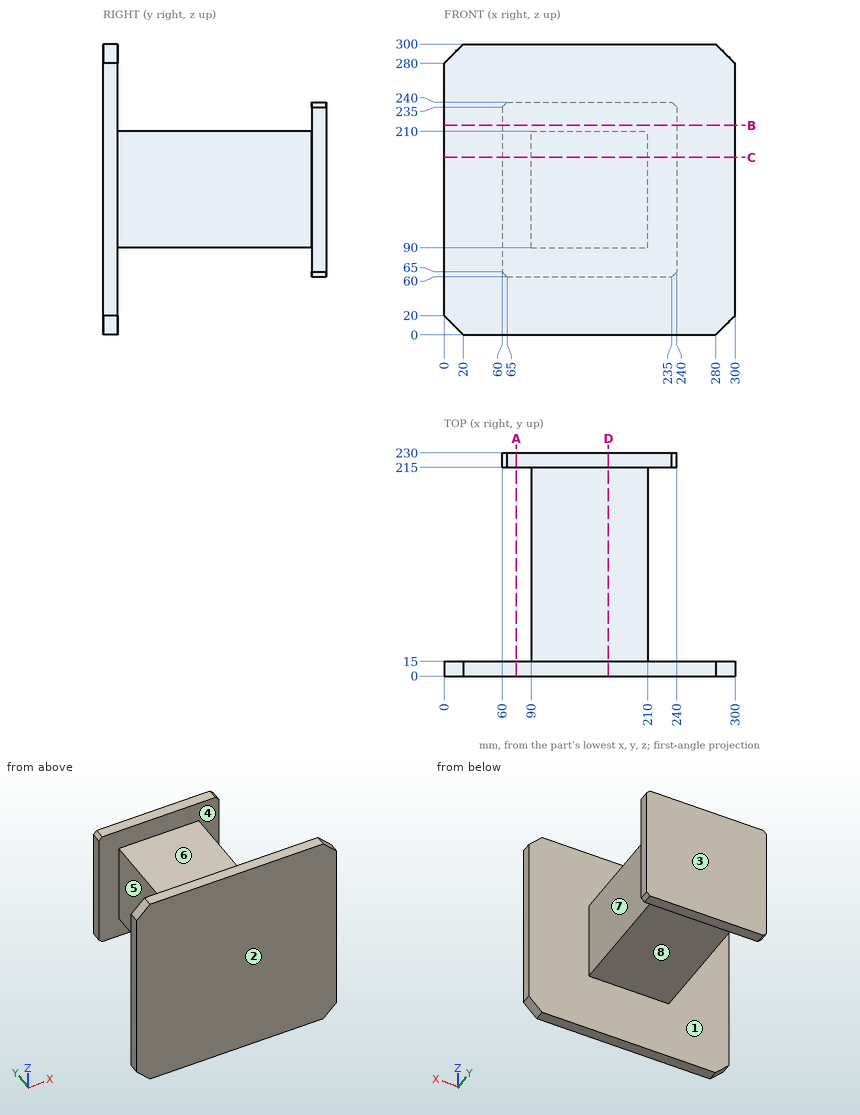
Print and shaded views of the part. All mm, measured from the part's lowest x, y and z. A direction names the side the tool comes from. Coordinates: 2 decimals unless noted, no trailing zeros. Order: outer loops, then holes, each group sorted by start corner. A loop starts at its lowest first (then second) coordinate and runs counter-clockwise, first axis right, second up. Notation, with made-up numbers: (42.25, 80.5) -> (60.25, 80.5) arc R25 ccw to (60.25, 102.5) -> close; hole circle Ø1 at (88.5, 73.5). An arc over 180 degrees is marked (long way). Answer as a JSON object with one key per item and string values. Group by question number.
1) Cut at B-B, the plane z = 216. Write the cut outline in (x, y).
2) Cut at C-C, the plane z = 183. Write the cut outline in (x, y).
3) Pull direction Y, two halves, no side cores. Call the marked faces 1, 2 and 3: +Y half, -Y half, draft (parallel to the pull), parting line (faces both ways), or undercut.
4) Flat gauge pins, fed straight in: pin 1 (3 mm diameter, centred on x = 190, y = 83.5, fed in from -Z); pin 2 (4.5 mm diameter, centred on y = 224.5, z = 182, fed in from +X); pin 3 (3 mm diameter, centred on y = 159, z = 203.5, fed in from +X); pin 4 (5 mm diameter, centred on x = 99.5, z = 88, fed in from -Y). Where does each tip first touch, or does it go through?
5) Cut at A-A, the plane x = 74.5. Write the cut outline in (y, z).
6) Drill centre lines: L1, parallel to Y at x = 211.5, z = 127; L2, parallel to Y at x = 41.5, z = 274; L3, parallel to X at y = 190, z = 136.5. Where is each one in solid material? Low to high.
7) Cut at D-D, the plane x = 169.5. Write the cut outline in (y, z), then the cut area to 3 significant figures.
8) Which spindle directions (+Z, -Z, +X, -X, +Y, -Y) get a long thin tool onto all of the face, cutting with end or side? Do the marked faces 4, 5, 6, 7 and 8. Say none if no direction does.
Check values:
{
 "1": {"outline": "(0, 0) -> (300, 0) -> (300, 15) -> (0, 15) -> close; (60, 215) -> (240, 215) -> (240, 230) -> (60, 230) -> close"},
 "2": {"outline": "(0, 0) -> (300, 0) -> (300, 15) -> (210, 15) -> (210, 215) -> (240, 215) -> (240, 230) -> (60, 230) -> (60, 215) -> (90, 215) -> (90, 15) -> (0, 15) -> close"},
 "3": {"face 1": "undercut", "face 2": "-Y half", "face 3": "+Y half"},
 "4": {"pin 1": "stops at z = 90", "pin 2": "stops at x = 240", "pin 3": "stops at x = 210", "pin 4": "stops at y = 0"},
 "5": {"outline": "(0, 0) -> (15, 0) -> (15, 300) -> (0, 300) -> close; (215, 60) -> (230, 60) -> (230, 240) -> (215, 240) -> close"},
 "6": {"L1": "y = 0 to 15, 215 to 230", "L2": "y = 0 to 15", "L3": "x = 90 to 210"},
 "7": {"outline": "(0, 0) -> (15, 0) -> (15, 90) -> (215, 90) -> (215, 60) -> (230, 60) -> (230, 240) -> (215, 240) -> (215, 210) -> (15, 210) -> (15, 300) -> (0, 300) -> close", "area": "31,200 mm²"},
 "8": {"face 4": "none", "face 5": "+Z, -Z, -X", "face 6": "+Z, +X, -X", "face 7": "+Z, -Z, +X", "face 8": "-Z, +X, -X"}
}
